from build123d import *

# Parameters (mm, degrees)
SKETCH_1_R                = 7
EXTRUDE_1_DEPTH           = 3
SKETCH_5_W                = 15
SKETCH_5_H                = 28
EXTRUDE_3_DEPTH           = 3
SKETCH_6_R                = 1.5
CUT_EXTRUDE_2_DEPTH       = 175.055428478
CHAMFER_1_SIZE            = 3.5
SKETCH_10_R               = 1.55
CUT_EXTRUDE_3_DEPTH       = 10
PATTERN_START             = -3
PATTERN_CURVE_1_OUTLINE_R = 1.55
PATTERN_CURVE_1_DEPTH     = 6
EXTRUDE_4_DEPTH           = 6
EXTRUDE_5_DEPTH           = 3
CHAMFER_2_SIZE            = 1
CHAMFER_3_SIZE            = 4.949606318
CHAMFER_3_SIZE_2          = 6
CHAMFER_3_SIZE_3          = 8.237528241
EXTRUDE_START             = 2
SKETCH_17_R               = 2.8
SKETCH_17_R_2             = 1.5
EXTRUDE_1_2_DEPTH         = 2
CHAMFER_4_SIZE            = 2
SKETCH1_R                 = 35.5
CUT_EXTRUDE1_DEPTH        = 10
BOSS_EXTRUDE1_DEPTH       = 6


# Read off the part's stored shape, not the designer's step: 曲线阵列1
with BuildPart() as part:
    # 草图1 → Extrude 1 (new, symmetric)
    with BuildSketch(Plane(origin=(0, 0, 0), x_dir=(0, 0, -1), z_dir=(1, 0, 0))):
        with BuildLine():
            ThreePointArc((102.937314742, -10), (106.138754414, -11.102344081), (107.982852519, -13.942006143))
            Line((107.982852519, -13.942006143), (123.580312189, -76.5))
            Line((123.580312189, -76.5), (144.192584776, -76.5))
            Line((144.192584776, -76.5), (126.405914526, -5.161562088))
            ThreePointArc((126.405914526, -5.161562088), (119.313229507, 5.760215072), (107, 10))
            Line((107, 10), (16, 10))
            ThreePointArc((16, 10), (11.149287499, 10.597149997), (6.588235294, 12.352941176))
            ThreePointArc((6.588235294, 12.352941176), (3.395498751, 13.581995002), (0, 14))
            Line((0, 14), (-18, 14))
            Line((-18, 14), (-18, 11))
            Line((-18, 11), (-13.388941598, -4.090995342))
            ThreePointArc((-13.388941598, -4.090995342), (-5.350452205, -12.937258643), (6.588235294, -12.352941176))
            ThreePointArc((6.588235294, -12.352941176), (11.149287499, -10.597149997), (16, -10))
            Line((16, -10), (102.937314742, -10))
        make_face()
        Circle(SKETCH_1_R, mode=Mode.SUBTRACT)
    extrude(amount=EXTRUDE_1_DEPTH, both=True)

    # 草图5 → 凸台-拉伸3 (add)
    with BuildSketch(Plane.XZ.offset(76.5)):
        with Locations((4.5, -134.192584776)):
            Rectangle(SKETCH_5_W, SKETCH_5_H)
    extrude(amount=EXTRUDE_3_DEPTH)

    # 草图6 → 切除-拉伸2 (cut, through all)
    with BuildSketch(Plane(origin=(0, -76.5, 0), x_dir=(1, 0, 0), z_dir=(0, 1, 0))):
        with Locations(Location((7.5, 143.192584776, 0), (0, 0, 270))):
            Circle(SKETCH_6_R)
        with Locations(Location((7.5, 125.192584776, 0), (0, 0, 90))):
            Circle(SKETCH_6_R)
    extrude(amount=-CUT_EXTRUDE_2_DEPTH, mode=Mode.SUBTRACT)

    # 倒角1
    chamfer_1_edges = [part.edges().sort_by_distance(p)[0] for p in [
        (12, -78, -148.192584776),
        (12, -78, -120.192584776),
    ]]
    chamfer(chamfer_1_edges, length=CHAMFER_1_SIZE)

    # 草图10 → 切除-拉伸3 (cut)
    with BuildSketch(Plane.ZY.offset(3)):
        with Locations((-25.5, 0)):
            Circle(SKETCH_10_R)
    extrude(amount=-CUT_EXTRUDE_3_DEPTH, mode=Mode.SUBTRACT)

    # 曲线阵列1 outline → 曲线阵列1 (cut)
    with BuildSketch(Plane.YZ.offset(PATTERN_START)):
        with Locations((-50.909555093, -127.506033962)):
            Circle(PATTERN_CURVE_1_OUTLINE_R)
        with Locations((-37.441286405, -124.148017428)):
            Circle(PATTERN_CURVE_1_OUTLINE_R)
        with Locations((-23.973017717, -120.790000895)):
            Circle(PATTERN_CURVE_1_OUTLINE_R)
        with Locations((-10.504749029, -117.431984361)):
            Circle(PATTERN_CURVE_1_OUTLINE_R)
        with Locations((-0.573099264, -108.725472335)):
            Circle(PATTERN_CURVE_1_OUTLINE_R)
        with Locations((0, -94.902906369)):
            Circle(PATTERN_CURVE_1_OUTLINE_R)
        with Locations((0, -81.022325095)):
            Circle(PATTERN_CURVE_1_OUTLINE_R)
        with Locations((0, -67.141743821)):
            Circle(PATTERN_CURVE_1_OUTLINE_R)
        with Locations((0, -53.261162547)):
            Circle(PATTERN_CURVE_1_OUTLINE_R)
        with Locations((0, -39.380581274)):
            Circle(PATTERN_CURVE_1_OUTLINE_R)
    extrude(amount=PATTERN_CURVE_1_DEPTH, mode=Mode.SUBTRACT)

    # 草图15 → 凸台-拉伸4 (add)
    with BuildSketch(Plane(origin=(3, 0, 0), x_dir=(0, 0, -1), z_dir=(1, 0, 0))):
        Polygon((-20.316390831, 14.441494507), (-19.448149943, 9.517455742), (-13.388941598, -4.090995342), (-18, 11), (-18, 14), (0, 14), align=None)
    extrude(amount=-EXTRUDE_4_DEPTH)

    # 草图16 → 凸台-拉伸5 (add, symmetric, along a direction that is not the sketch's normal)
    with BuildSketch(Plane(origin=(0, 26.950685529, -108.093295667), x_dir=(-1, 0, 0), z_dir=(0, 0.2419218955996646, -0.9702957262759974))):
        Polygon((-12, -106.691747545), (-3, -88.691747545), (-3, -106.691747545), align=None)
    extrude(amount=EXTRUDE_5_DEPTH, dir=(0, 0, -1), both=True)

    # 倒角2
    chamfer_2_edges = [part.edges().sort_by_distance(p)[0] for p in [
        (3, -76.5, -140.539516629),
        (3, -76.5, -127.233380336),
    ]]
    chamfer(chamfer_2_edges, length=CHAMFER_2_SIZE)

    # 倒角3
    # the kernel refuses this chamfer: 8.237528241, 6, 4.949606318 mm, written as the material it adds along each edge
    with BuildSketch(Plane(origin=(19.430097928, -76.5, -123.580312189), x_dir=(0, -0.04051695164362419, 0.9991788511720553), z_dir=(-1, 0, 0))) as chamfer_3_piece_1_section:
        Polygon((CHAMFER_3_SIZE * 0.999178851168, CHAMFER_3_SIZE * 0.0405169516434), (CHAMFER_3_SIZE_2 * 0.202409816697, CHAMFER_3_SIZE_2 * 0.979300906823), (0, 0), align=None)
    chamfer_3_piece_1 = extrude(amount=22.430097928, mode=Mode.PRIVATE)
    chamfer_3_piece_1 = split(chamfer_3_piece_1, bisect_by=Plane(origin=(3, -73.046454267, -121.751433379), z_dir=(-1, 0, 0)), keep=Keep.TOP, mode=Mode.PRIVATE)
    chamfer_3_piece_1 = split(chamfer_3_piece_1, bisect_by=Plane(origin=(1.773227133, -73.046454267, -120.192584776), z_dir=(0, 0, -1)), keep=Keep.TOP, mode=Mode.PRIVATE)
    add(chamfer_3_piece_1)
    with BuildSketch(Plane(origin=(19.430097928, -76.5, -123.580312189), x_dir=(0, -0.04051695164362419, 0.9991788511720553), z_dir=(-1, 0, 0))) as chamfer_3_piece_2_section:
        Polygon((CHAMFER_3_SIZE * 0.999178851168, CHAMFER_3_SIZE * 0.0405169516434), (CHAMFER_3_SIZE_2 * 0.202409816697, CHAMFER_3_SIZE_2 * 0.979300906823), (0, 0), align=None)
    chamfer_3_piece_2 = extrude(amount=22.430097928, mode=Mode.PRIVATE)
    chamfer_3_piece_2 = split(chamfer_3_piece_2, bisect_by=Plane(origin=(3.335429121, -76.170858242, -120.192584776), z_dir=(0, 0, -1)), keep=Keep.TOP, mode=Mode.PRIVATE)
    chamfer_3_piece_2 = split(chamfer_3_piece_2, bisect_by=Plane(origin=(3.503143682, -76.003143682, -121.845416354), z_dir=(-0.7071067811865476, -0.7071067811865476, 0)), keep=Keep.TOP, mode=Mode.PRIVATE)
    add(chamfer_3_piece_2)
    with BuildSketch(Plane(origin=(-3, -76.5, -144.192584776), x_dir=(4.057410477830116e-15, -0.037354428652640735, -0.9993020797837033), z_dir=(1, 0, 0))) as chamfer_3_piece_3_section:
        Polygon((CHAMFER_3_SIZE_2 * 0.999302079784, CHAMFER_3_SIZE_2 * 0.0373544286526), (-CHAMFER_3_SIZE_3 * 0.277997895888, CHAMFER_3_SIZE_3 * 0.960581683052), (0, 0), align=None)
    chamfer_3_piece_3 = extrude(amount=28.304139536, mode=Mode.PRIVATE)
    chamfer_3_piece_3 = split(chamfer_3_piece_3, bisect_by=Plane(origin=(0.670769547, -73.170769547, -145.630202159), z_dir=(-0.7071067811865476, -0.7071067811865476, 0)), keep=Keep.TOP, mode=Mode.PRIVATE)
    chamfer_3_piece_3 = split(chamfer_3_piece_3, bisect_by=Plane(origin=(-0.598503723, -74.440042816, -148.192584776), z_dir=(0, 0, 1)), keep=Keep.TOP, mode=Mode.PRIVATE)
    add(chamfer_3_piece_3)
    with BuildSketch(Plane(origin=(-3, -76.5, -144.192584776), x_dir=(4.057410477830116e-15, -0.037354428652640735, -0.9993020797837033), z_dir=(1, 0, 0))) as chamfer_3_piece_4_section:
        Polygon((CHAMFER_3_SIZE_2 * 0.999302079784, CHAMFER_3_SIZE_2 * 0.0373544286526), (-CHAMFER_3_SIZE_3 * 0.277997895888, CHAMFER_3_SIZE_3 * 0.960581683052), (0, 0), align=None)
    chamfer_3_piece_4 = extrude(amount=28.304139536, mode=Mode.PRIVATE)
    chamfer_3_piece_4 = split(chamfer_3_piece_4, bisect_by=Plane(origin=(3, -72.000472632, -144.373314083), z_dir=(-1, 0, 0)), keep=Keep.TOP, mode=Mode.PRIVATE)
    chamfer_3_piece_4 = split(chamfer_3_piece_4, bisect_by=Plane(origin=(1.258880845, -72.000472632, -148.192584776), z_dir=(0, 0, 1)), keep=Keep.TOP, mode=Mode.PRIVATE)
    add(chamfer_3_piece_4)

    # 草图17 → Extrude 1 2 (add)
    # profile 1 of 2: a face of its own
    with BuildSketch(Plane(origin=(0, -76.5, 0), x_dir=(1, 0, 0), z_dir=(0, 1, 0)).offset(EXTRUDE_START)):
        with Locations((7.5, 125.192584776)):
            Circle(SKETCH_17_R)
        with Locations((7.5, 125.192584776)):
            Circle(SKETCH_17_R_2, mode=Mode.SUBTRACT)
    # profile 2 of 2: a face of its own
    with BuildSketch(Plane(origin=(0, -76.5, 0), x_dir=(1, 0, 0), z_dir=(0, 1, 0)).offset(EXTRUDE_START)):
        with Locations((7.5, 143.192584776)):
            Circle(SKETCH_17_R)
        with Locations((7.5, 143.192584776)):
            Circle(SKETCH_17_R_2, mode=Mode.SUBTRACT)
    extrude(amount=-EXTRUDE_1_2_DEPTH)

    # 倒角4
    # the kernel refuses this chamfer: 2 mm, written as the material it adds along each edge
    with BuildSketch(Plane(origin=(7.5, -76.5, -125.192584776), x_dir=(1, 0, 0), z_dir=(0, 0, 1))) as chamfer_4_piece_1_section:
        Polygon((2.8 + CHAMFER_4_SIZE, 0), (2.8, CHAMFER_4_SIZE), (2.8, 0), align=None)
    chamfer_4_piece_1 = revolve(axis=Axis((7.5, -76.5, -125.192584776), (0, 1, 0)), mode=Mode.PRIVATE)
    chamfer_4_piece_1 = split(chamfer_4_piece_1, bisect_by=Plane(origin=(8.598627061, -75.553822664, -120.291211837), z_dir=(-0.7071067811865476, 0, -0.7071067811865476)), keep=Keep.TOP, mode=Mode.PRIVATE)
    chamfer_4_piece_1 = split(chamfer_4_piece_1, bisect_by=Plane(origin=(12, -75.553822664, -125.192584776), z_dir=(-1, 0, 0)), keep=Keep.TOP, mode=Mode.PRIVATE)
    chamfer_4_piece_1 = split(chamfer_4_piece_1, bisect_by=Plane(origin=(3.697254122, -74.5, -125.192584776), z_dir=(0, -1, 0)), keep=Keep.TOP, mode=Mode.PRIVATE)
    add(chamfer_4_piece_1)
    with BuildSketch(Plane(origin=(7.5, -76.5, -143.192584776), x_dir=(1, 0, 0), z_dir=(0, 0, 1))) as chamfer_4_piece_2_section:
        Polygon((2.8 + CHAMFER_4_SIZE, 0), (2.8, CHAMFER_4_SIZE), (2.8, 0), align=None)
    chamfer_4_piece_2 = revolve(axis=Axis((7.5, -76.5, -143.192584776), (0, 1, 0)), mode=Mode.PRIVATE)
    chamfer_4_piece_2 = split(chamfer_4_piece_2, bisect_by=Plane(origin=(8.598627061, -75.553822664, -148.093957715), z_dir=(-0.7071067811865476, 0, 0.7071067811865476)), keep=Keep.TOP, mode=Mode.PRIVATE)
    chamfer_4_piece_2 = split(chamfer_4_piece_2, bisect_by=Plane(origin=(12, -75.553822664, -143.192584776), z_dir=(-1, 0, 0)), keep=Keep.TOP, mode=Mode.PRIVATE)
    chamfer_4_piece_2 = split(chamfer_4_piece_2, bisect_by=Plane(origin=(3.697254121, -74.5, -143.192584776), z_dir=(0, -1, 0)), keep=Keep.TOP, mode=Mode.PRIVATE)
    add(chamfer_4_piece_2)

    # Sketch1 → Cut-Extrude1 (cut)
    with BuildSketch(Plane(origin=(3, 0, 0), x_dir=(0, 0, -1), z_dir=(1, 0, 0))):
        with Locations((86.954808596, -52.5)):
            Circle(SKETCH1_R)
    extrude(amount=-CUT_EXTRUDE1_DEPTH, mode=Mode.SUBTRACT)

    # Sketch2 → Boss-Extrude1 (add)
    with BuildSketch(Plane(origin=(3, 0, 0), x_dir=(0, 0, -1), z_dir=(1, 0, 0))):
        Polygon((126.405914526, -5.161562088), (134.122760953, -17.511097881), (141.602601038, -47.511097881), (140.567007759, -61.958604825), align=None)
    extrude(amount=-BOSS_EXTRUDE1_DEPTH)


solid = part.part
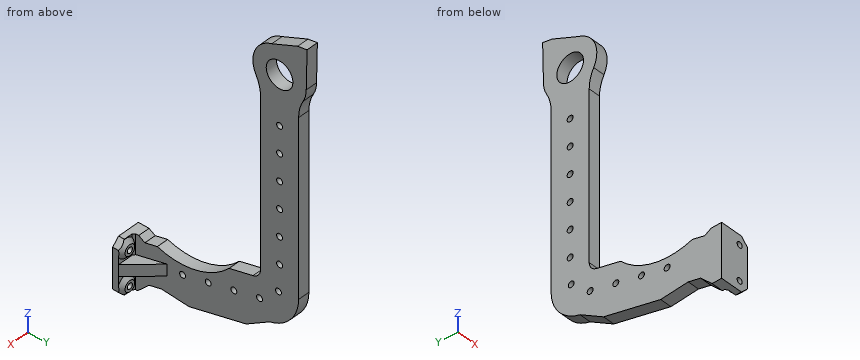
Can you work these out from the model? Positions are in its coordinate system, mm. Give positions to 0.01 mm unless a question says otherwise; leave off trailing zeros. Loops run counter-clockwise (first coordinate to the right, second up) from the corner with the lowest first, then second, coordinate; pieces in that order, holes last. Notation, with made-up numbers: M -32,32.5 L -20,32.5 A30 ccw -20,59.5 Z; hole C 85.5,59.5 d8. An arc over 180 degrees is marked long. One line per item, written item: value. Start each with the question number.
1) If we section it at D-D, the plane z = -57: Write out the boundary of the cut face in (x, y).
2) I'm going to push flat-ended pins straight in: pin 1 (6.5 mm diameter, centred on x = -0.5, z = -63, fed in from -Y); pin 2 (1.7 mm diameter, centred on x = 7, z = -126.5, fed in from +Y); pin 3 (3 mm diameter, centred on x = 1, z = 1.5, fed in from +Y). Where does each tip first touch, or does it pass through?
3) If I drill on line 1 (Z direction, x = 7.5, y = -77.9); line 2 (Y direction, x = -0.6, z = 0); line 3 (Y direction, x = 1.5, z = -18), over which ranges is the centre line in solid material (lowest first)? Write a range as [from, to].
4) If we section it at C-C, the plane x = -1: Give the number of separate pieces and of enclosed holes in the cut face, and give its area (3 significant figures).
5) If we section it at B-B, the plane y = -66: Write out the boundary of the cut face in (x, z).
6) If we section it at A-A, the plane z = -25.5: Write out the boundary of the cut face in (x, y), and give its area (3 significant figures).
Completed:
1. outline: M -3,-10 L 3,-10 L 3,10 L -3,10 Z
2. pin 1: stops at y = -10
2. pin 2: stops at y = -74.5
2. pin 3: stops at y = 14.07
3. line 1: z = [-148.19, -144.69], [-141.69, -126.69], [-123.69, -120.19]
3. line 2: y = [-14, -7], [7, 14]
3. line 3: y = [-10, 10]
4. separate pieces: 1
4. enclosed holes: 12
4. area: 4,230 mm^2
5. outline: M -3,-141.57 L 3,-141.57 L 3,-134.27 L 6.55,-134.27 L 6.55,-128.27 L 3,-128.27 L 3,-120.96 L -3,-120.96 Z
6. outline: M -3,-10 L 3,-10 L 3,-1.55 L -3,-1.55 Z; M -3,1.55 L 3,1.55 L 3,10 L -3,10 Z
6. area: 101 mm^2
